from build123d import *

# Parameters (mm, degrees)
EXTRUDE_1_DEPTH = 3


with BuildPart() as part:
    # 草图2 → 凸台-拉伸1 (new body)
    with BuildSketch(Plane.XY):
        with BuildLine():
            Line((2.047890023, 48.855305477), (8, 48.855305477))
            Line((8, 48.855305477), (8, 51.855305477))
            Line((8, 51.855305477), (16, 51.855305477))
            Line((16, 51.855305477), (16, 19.855305477))
            Line((16, 19.855305477), (8, 19.855305477))
            Line((8, 19.855305477), (8, 16.855305477))
            Line((8, 16.855305477), (0.390512484, 16.855305477))
            ThreePointArc((0.390512484, 16.855305477), (0, 19.905305477), (-0.390512484, 16.855305477))
            Line((-0.390512484, 16.855305477), (-8, 16.855305477))
            Line((-8, 16.855305477), (-8, 19.855305477))
            Line((-8, 19.855305477), (-16, 19.855305477))
            Line((-16, 19.855305477), (-16, 51.855305477))
            Line((-16, 51.855305477), (-8, 51.855305477))
            Line((-8, 51.855305477), (-8, 48.855305477))
            Line((-8, 48.855305477), (-2.047890023, 48.855305477))
            Line((-2.047890023, 48.855305477), (-2.047890023, 43.855305477))
            Line((-2.047890023, 43.855305477), (-4, 43.855305477))
            Line((-4, 43.855305477), (-4, 40.855305477))
            Line((-4, 40.855305477), (-2, 40.855305477))
            Line((-2, 40.855305477), (-2, 36.855305477))
            Line((-2, 36.855305477), (2, 36.855305477))
            Line((2, 36.855305477), (2, 40.855305477))
            Line((2, 40.855305477), (4, 40.855305477))
            Line((4, 40.855305477), (4, 43.855305477))
            Line((4, 43.855305477), (2.047890023, 43.855305477))
            Line((2.047890023, 43.855305477), (2.047890023, 48.855305477))
        make_face()
    extrude(amount=EXTRUDE_1_DEPTH)


solid = part.part
Verification items for the finished model (mm, model axes). A direction names the side the tool comes from. Give positions to 0.01 mm unless a question says otherwise; leave off trailing zeros. Loops run counter-clockwise (first coordinate to the right, second up) from the corner with the lowest first, then second, coordinate; pieces in that order, holes last.
1. Cross-section at A-A on y = 42. Record the cut outline in (x, z), and give its area (3 significant figures).
Derived:
outline: (-16, 0) - (-4, 0) - (-4, 3) - (-16, 3) - close; (4, 0) - (16, 0) - (16, 3) - (4, 3) - close
area: 72.0 mm2
2. Cross-section at B-B on x = 1. Record the cut outline in (y, z).
Derived:
outline: (16.86, 0) - (17.17, 0) - (17.17, 3) - (16.86, 3) - close; (19.54, 0) - (36.86, 0) - (36.86, 3) - (19.54, 3) - close
3. Go/stop test with flat-tipped pins: P1, Ø1.5, axis at x = 12.5, z = 1.5, coming from the -Y side; P2, Ø0.9, axis at x = 6.5, z = 1.5, coming from the +Y side; P3, Ø0.9, axis at y = 18, z = 1, coming from the +X side. Record where each tip stops, or that it passes through.
Derived:
P1: stops at y = 19.86
P2: stops at y = 48.86
P3: stops at x = 8
4. Cross-section at C-C on z = 2.25. Record the cut outline in (x, y).
Derived:
outline: (-16, 19.86) - (-8, 19.86) - (-8, 16.86) - (-0.39, 16.86) arc R1.55 cw (long way) to (0.39, 16.86) - (8, 16.86) - (8, 19.86) - (16, 19.86) - (16, 51.86) - (8, 51.86) - (8, 48.86) - (2.05, 48.86) - (2.05, 43.86) - (4, 43.86) - (4, 40.86) - (2, 40.86) - (2, 36.86) - (-2, 36.86) - (-2, 40.86) - (-4, 40.86) - (-4, 43.86) - (-2.05, 43.86) - (-2.05, 48.86) - (-8, 48.86) - (-8, 51.86) - (-16, 51.86) - close
5. Material ranges on probe 1 along X at (y, z) = (49, 0.75); probe 2 along X at (y, z) = (47.5, 1.7); probe 3 along Y at (x, z) = (3, 2.3), recorded low to high.
Derived:
probe 1: x = -16 to -8, 8 to 16
probe 2: x = -16 to -2.05, 2.05 to 16
probe 3: y = 16.86 to 40.86, 43.86 to 48.86
6. Cross-section at D-D on x = -9.5. Record the cut outline in (y, z), and give its area (3 significant figures).
Derived:
outline: (19.86, 0) - (51.86, 0) - (51.86, 3) - (19.86, 3) - close
area: 96.0 mm2
7. Release check for a two-part mould opening along Y. For faces 1 (the flat face through (12, 51.855, 1)), 2 (the flat face through (8, 18, 1)), 3 (the flat face through (-4, 42, 1)) record: +Y half, -Y half, draft (parallel to the pull), parting line (faces both ways), or undercut.
Derived:
face 1: +Y half
face 2: draft
face 3: undercut
8. Tool access check on faces 4 (the flat face through (12, 19.855, 1)), 5 (the flat face through (-8, 18, 1)), 6 (the flat face through (3, 40.855, 1)), 7 (the flat face through (2.048, 46, 1)), 8 (the flat face through (0, 35, 3)). Record the directions out of +Z, -Z, +X, -X, +Y, -Y that give a thin tool (end or side, any length) a straight path to the whole face; none if there is none.
Derived:
face 4: +Z, -Z, +X, -Y
face 5: +Z, -Z, -X, -Y
face 6: +Z, -Z
face 7: +Z, -Z, +Y
face 8: +Z, +X, -X, +Y, -Y
